from build123d import *

# Parameters (mm, degrees)
F1_DEPTH = 25.4
F0_W     = 12.7
F0_H     = 31.75
F2_DEPTH = 25.4
F4_DEPTH = 12.7
F6_R     = 38.1
F7_DEPTH = 25.4
F8_DEPTH = 12.7


# Not quite as in the source:
# - a feature names something its author has since deleted; it is built from what else it names


with BuildPart() as f1:
    # F0 (on Top) → F1 (new body)
    with BuildSketch(Plane.XY):
        with BuildLine():
            Line((-76.2, 209.55), (-76.2, 0))
            Line((-76.2, 0), (76.2, 0))
            Line((76.2, 0), (76.2, 209.55))
            ThreePointArc((76.2, 209.55), (74.3401280605, 214.0401280605), (69.85, 215.9))
            Line((69.85, 215.9), (31.75, 215.9))
            ThreePointArc((31.75, 215.9), (27.2598719395, 217.7598719395), (25.4, 222.25))
            Line((25.4, 222.25), (12.7, 222.25))
            Line((12.7, 222.25), (12.7, 215.9))
            ThreePointArc((12.7, 215.9), (0, 203.2), (-12.7, 215.9))
            Line((-12.7, 215.9), (-12.7, 222.25))
            Line((-12.7, 222.25), (-25.4, 222.25))
            ThreePointArc((-25.4, 222.25), (-27.2598719395, 217.7598719395), (-31.75, 215.9))
            Line((-31.75, 215.9), (-69.85, 215.9))
            ThreePointArc((-69.85, 215.9), (-74.3401280605, 214.0401280605), (-76.2, 209.55))
        make_face()
        with BuildLine():
            Line((-50.8, 101.6), (-50.8, 177.8))
            ThreePointArc((-50.8, 177.8), (-38.1, 190.5), (-25.4, 177.8))
            Line((-25.4, 177.8), (-25.4, 101.6))
            ThreePointArc((-25.4, 101.6), (-38.1, 88.9), (-50.8, 101.6))
        make_face(mode=Mode.SUBTRACT)
        with BuildLine():
            Line((25.4, 101.6), (25.4, 177.8))
            ThreePointArc((25.4, 177.8), (38.1, 190.5), (50.8, 177.8))
            Line((50.8, 177.8), (50.8, 101.6))
            ThreePointArc((50.8, 101.6), (38.1, 88.9), (25.4, 101.6))
        make_face(mode=Mode.SUBTRACT)
    extrude(amount=F1_DEPTH)

    # F0 (on Top) → F2 (join)
    with BuildSketch(Plane.XY):
        with Locations((-19.05, 238.125)):
            Rectangle(F0_W, F0_H)
        with Locations((19.05, 238.125)):
            Rectangle(F0_W, F0_H)
    extrude(amount=F2_DEPTH)

    # F3 (on Right) → F4 (join, symmetric)
    with BuildSketch(Plane.YZ):
        Polygon((25.4, 76.2), (25.4, 25.4), (63.5, 25.4), align=None)
    extrude(amount=F4_DEPTH, both=True)

    # F6 (on Front) → F7 (join)
    with BuildSketch(Plane.XZ):
        with BuildLine():
            Line((-76.2, 25.4), (76.2, 25.4))
            Line((76.2, 25.4), (76.2, 127))
            ThreePointArc((76.2, 127), (53.8815367264, 180.8815367264), (0, 203.2))
            ThreePointArc((0, 203.2), (-53.8815367264, 180.8815367264), (-76.2, 127))
            Line((-76.2, 127), (-76.2, 25.4))
        make_face()
        with Locations((0, 127)):
            Circle(F6_R, mode=Mode.SUBTRACT)
    extrude(amount=-F7_DEPTH)

    # F0 (on Top) → F8 (join)
    with BuildSketch(Plane.XY):
        with BuildLine():
            Line((-12.7, 254), (-12.7, 222.25))
            Line((-12.7, 222.25), (-12.7, 215.9))
            ThreePointArc((-12.7, 215.9), (0, 203.2), (12.7, 215.9))
            Line((12.7, 215.9), (12.7, 222.25))
            Line((12.7, 222.25), (12.7, 254))
            Line((12.7, 254), (-12.7, 254))
        make_face()
    extrude(amount=F8_DEPTH)


solid = f1.part
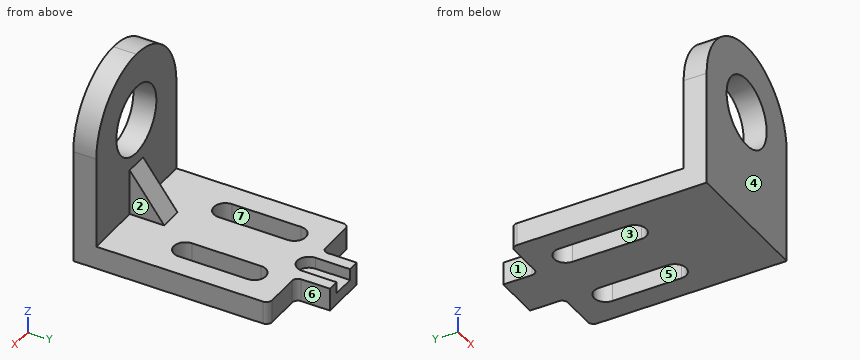
Source: CAD feature listing. Evaluate the final solid. Frame: model axes, mm. Face numbers are marked on the shaded views. A direction names the side the tool comes from. Round coordinates to 2 decimals unless told otherwise and drop trailing zeros. Loops run counter-clockwise (first coordinate to the right, second up) from the corner with the lowest first, then second, coordinate; pieces in that order, holes last. Notation, with made-up numbers: (32, 13) -> (90, 13) arc R24 ccw to (90, 42) -> close; hole circle Ø5 at (75.25, -19). An arc over 180 degrees is marked (long way). Answer as a JSON object with one key per item and string values. Group by question number.
Q1. Mould query, pull axis X, two halves, no side actions, for the marked faces 4, 5, 6 and 7. Classes: pulls with the +X half, pulls with the -X half, needs draft (parallel to the pull), parting line crosses it, or undercut.
Q2. Section query C-C (x = -35). Output: boundary loops of the cut face in (y, z), plus the area to 3 significant figures.
Q3. Section query A-A (y = 134.5). Output: boundary loops of the cut face in (x, z).
Q4. Ray query, line 1 (Z direction, x = 55.5, y = 132); line 2 (Z direction, x = 5.5, y = 214). Return the intervals inside material, ascending. Write a range as from..to.
Q5. Contact query for flat-ended pins moving along their axis: P1, Ø8, axis at x = -23, z = 103, coming from the +Y side; P2, Ø14, axis at y = 236.5, z = 21, coming from the +X side; P3, Ø12.5, axis at x = -45.5, z = 8, coming from the +Y side; P4, Ø12, axis at x = 29.5, z = 98.5, coming from the +Y side. Output: stop coordinate, or through.
Q6. Section query D-D (y = 229). Output: boundary loops of the cut face in (x, z), plus the area to 3 significant figures.
Q7. Access query for the marked faces 1, 2 and 3. Directions: +Z, -Z, +X, -X, +Y, -Y. A direction counts if a zero-diameter tool reaches every point of the face in a straight line with its end or side. Return the directions, or none.
Q8. Section query B-B (z = 143.5). Output: boundary loops of the cut face in (x, y).
Completed:
{
 "1": {"face 4": "needs draft", "face 5": "undercut", "face 6": "pulls with the +X half", "face 7": "undercut"},
 "2": {"outline": "(0, 0) -> (89.28, 0) -> (89.28, 25.4) -> (25.4, 25.4) -> (25.4, 111.95) -> (0, 111.95) -> close; (0, 142.05) -> (25.4, 142.05) -> (25.4, 194.69) -> (0, 194.69) -> close; (190.12, 0) -> (215.9, 0) -> (215.9, 25.4) -> (190.12, 25.4) -> close", "area": "6,460 mm²"},
 "3": {"outline": "(-76.2, 0) -> (-50.8, 0) -> (-50.8, 25.4) -> (-76.2, 25.4) -> close; (-25.4, 0) -> (25.4, 0) -> (25.4, 25.4) -> (-25.4, 25.4) -> close; (50.8, 0) -> (76.2, 0) -> (76.2, 25.4) -> (50.8, 25.4) -> close"},
 "4": {"line 1": "0..25.4", "line 2": "0..12.7"},
 "5": {"P1": "through", "P2": "x = 25.4", "P3": "y = 215.9", "P4": "y = 25.4"},
 "6": {"outline": "(-25.4, 0) -> (25.4, 0) -> (25.4, 25.4) -> (12.7, 25.4) -> (12.7, 12.7) -> (-12.7, 12.7) -> (-12.7, 25.4) -> (-25.4, 25.4) -> close", "area": "968 mm²"},
 "7": {"face 1": "+Z, -Z, -X, +Y", "face 2": "+Z, +X, +Y", "face 3": "+Z, -Z"},
 "8": {"outline": "(-74.39, 0) -> (-34.34, 0) -> (-34.34, 25.4) -> (-74.39, 25.4) -> close; (34.34, 0) -> (74.39, 0) -> (74.39, 25.4) -> (34.34, 25.4) -> close"}
}
